from build123d import *

# Parameters (mm, degrees)
F1_DEPTH = 60.96
F2_W     = 15.180191
F2_H     = 51.094524
F3_DEPTH = 12.7
F4_R     = 12.7
F5_R     = 6.35
F6_DEPTH = 50.8


with BuildPart() as f1:
    # F0 (on Front) → F1 (new body)
    with BuildSketch(Plane.XZ):
        with BuildLine():
            Line((-66.034004, 15.106326), (-68.026364, 0))
            Line((-68.026364, 0), (65.327539, 0))
            Line((65.327539, 0), (65.327539, 53.066271))
            ThreePointArc((65.327539, 53.066271), (62.7831, 58.149598), (57.18889, 59.159155))
            Line((57.18889, 59.159155), (-57.020338, 25.631483))
            ThreePointArc((-57.020338, 25.631483), (-63.089174, 21.706593), (-66.034004, 15.106326))
        make_face()
    extrude(amount=F1_DEPTH)

    # F2 (on face) → F3 (cut)
    with BuildSketch(Plane(origin=(-11.451568, 0, 39.008815), x_dir=(0.959509, 0, 0.281677), z_dir=(-0.281677, 0, 0.959509))):
        with Locations((38.148094, -31.626057)):
            Rectangle(F2_W, F2_H)
    extrude(amount=-F3_DEPTH, mode=Mode.SUBTRACT)

    # F4
    f4_edges = [f1.edges().sort_by_distance(p)[0] for p in [
        (-68.026364, -30.48, 0),
    ]]
    fillet(f4_edges, radius=F4_R)

    # F5 (on face) → F6 (cut)
    with BuildSketch(Plane.YZ.offset(65.327539)):
        with Locations((-52.006502, 12.382501)):
            Circle(F5_R)
        with Locations((-31.813502, 12.382501)):
            Circle(F5_R)
        with Locations((-12.192, 12.382501)):
            Circle(F5_R)
    extrude(amount=-F6_DEPTH, mode=Mode.SUBTRACT)


solid = f1.part
Can you work these out from the model? Positions are in its coordinate system, mm. A direction names the side the tool comes from. Give positions to 0.01 mm unless a question says otherwise; leave off trailing zeros. Loops run counter-clockwise (first coordinate to the right, second up) from the corner with the lowest first, then second, coordinate; pieces in that order, holes last. Notation, with made-up numbers: (43, 83.5) -> (99, 83.5) arc R24 ccw to (99, 109.5) -> close; hole circle Ø7 at (3, -29). An arc over 180 degrees is marked (long way). Return JSON: item names as keys, results as strings.
Q1. I want a section at C-C, the plane x = 20. List the corners of the cut face in (y, z) for me.
Checks:
{"outline": "(-60.96, 0) -> (0, 0) -> (0, 48.24) -> (-6.08, 48.24) -> (-6.08, 40.36) -> (-57.17, 40.36) -> (-57.17, 48.24) -> (-60.96, 48.24) -> close; hole circle Ø12.7 at (-52.01, 12.38); hole circle Ø12.7 at (-31.81, 12.38); hole circle Ø12.7 at (-12.19, 12.38)"}
Q2. I want a section at D-D, the plane z = 50.5. List the corners of the cut face in (x, y) for me, then the cut area to 3 significant figures.
Checks:
{"outline": "(27.69, -60.96) -> (65.33, -60.96) -> (65.33, 0) -> (27.69, 0) -> (27.69, -6.08) -> (32.84, -6.08) -> (32.84, -57.17) -> (27.69, -57.17) -> close", "area": "2,030 mm2"}
Q3. On a 3-axis mill with a long thin cutter (end or side, diameter ignored), from which of +Z, -Z, +X, -X, +Y, -Y can I reach the whole of each face in a straight line? I mean faces 1 (the face through (27, -6.079, 44)), 2 (the face through (13, 0, 24)), 3 (the face through (19.633, -31.984, 41.609)), 4 (the face through (14.528, -12, 12)), 5 (the face through (-63.022, -30.053, 21.784)). Say none if no direction works.
Checks:
{"face 1": "none", "face 2": "+Z, -Z, +X, -X, +Y", "face 3": "+Z", "face 4": "+X", "face 5": "+Z, -X, +Y, -Y"}
Q4. We'd pull the mould along X, two halves only. Please class faces 6 (the face through (62.85, -30.05, 58.1)), 7 (the face through (40.28, -8.78, 17.74)), 8 (the face through (28.63, -31.27, 37.54)): released by +X, released by -X, zero draft, split by the parting line, or undercut.
Checks:
{"face 6": "split by the parting line", "face 7": "zero draft", "face 8": "undercut"}
Q5. I want a section at A-A, the plane y = -42. List the corners of the cut face in (x, z) for me.
Checks:
{"outline": "(-66.13, 14.36) arc R12.7 ccw to (-53.54, 0) -> (65.33, 0) -> (65.33, 53.07) arc R6.35 ccw to (57.19, 59.16) -> (32.43, 51.89) -> (36.01, 39.71) -> (21.45, 35.43) -> (17.87, 47.62) -> (-57.02, 25.63) arc R12.7 ccw to (-66.03, 15.11) -> close"}
Q6. I want a section at B-B, the plane z = 37.5. List the corners of the cut face in (x, y) for me.
Checks:
{"outline": "(-16.59, -60.96) -> (65.33, -60.96) -> (65.33, 0) -> (-16.59, 0) -> close; hole (20.84, -57.17) -> (28.5, -57.17) -> (28.5, -6.08) -> (20.84, -6.08) -> close"}
Q7. I need wall thicknesses on probe 1 along Z at (x, y) = (29, -53); probe 2 along Y at (x, z) = (19.5, 11); probe 3 along X at (y, z) = (-44, 10.5). Which ranges of each line are inside material? Lowest first, please.
Checks:
{"probe 1": "z = 0 to 6.11, 18.65 to 37.65", "probe 2": "y = -60.96 to -58.2, -45.81 to -38.01, -25.62 to -18.39, -5.99 to 0", "probe 3": "x = -66.05 to 65.33"}
Q8. For pin 1 Ø7.5 at (y, z) = (-12.19, 12.38) entering from +X; pin 2 Ø1.5 at (x, y) = (31, -36) entering from +Z, each with a flat end and sliding along its axis, tell me the tip position at first contact or that it passes through.
Checks:
{"pin 1": "stops at x = 14.53", "pin 2": "stops at z = 38.46"}
